```python
from build123d import *

# Parameters (mm, degrees)
BOSS_EXTRUDE1_DEPTH = 2.5
SKETCH2_R           = 1.5
CUT_EXTRUDE1_DEPTH  = 10
SKETCH3_R           = 4.25
SKETCH3_R_2         = 2.75
BOSS_EXTRUDE2_DEPTH = 3.5
SKETCH4_R           = 3.75
SKETCH4_R_2         = 3.25
BOSS_EXTRUDE3_DEPTH = 0.5


with BuildPart() as part:
    # Sketch1 → Boss-Extrude1 (new body)
    with BuildSketch(Plane(origin=(0, 0, 0), x_dir=(1, 0, 0), z_dir=(0, 1, 0))):
        with BuildLine():
            Line((10, -4), (17.506131517, -2.448230154))
            ThreePointArc((17.506131517, -2.448230154), (19.5, 0), (17.506131517, 2.448230154))
            Line((17.506131517, 2.448230154), (10, 4))
            Line((10, 4), (3.774917218, 4))
            ThreePointArc((3.774917218, 4), (0, 5.5), (-3.774917218, 4))
            Line((-3.774917218, 4), (-10, 4))
            Line((-10, 4), (-17.506131517, 2.448230154))
            ThreePointArc((-17.506131517, 2.448230154), (-19.5, 0), (-17.506131517, -2.448230154))
            Line((-17.506131517, -2.448230154), (-10, -4))
            Line((-10, -4), (-3.774917218, -4))
            ThreePointArc((-3.774917218, -4), (0, -5.5), (3.774917218, -4))
            Line((3.774917218, -4), (10, -4))
        make_face()
    extrude(amount=BOSS_EXTRUDE1_DEPTH)

    # Sketch2 → Cut-Extrude1 (cut)
    with BuildSketch(Plane(origin=(0, 2.5, 0), x_dir=(1, 0, 0), z_dir=(0, 1, 0))):
        with Locations(Location((0, 0, 0), (0, 0, 270))):
            Circle(SKETCH2_R)
    extrude(amount=-CUT_EXTRUDE1_DEPTH, mode=Mode.SUBTRACT)

    # Sketch3 → Boss-Extrude2 (add)
    with BuildSketch(Plane(origin=(0, 2.5, 0), x_dir=(1, 0, 0), z_dir=(0, 1, 0))):
        with Locations(Location((0, 0, 0), (0, 0, 270))):
            Circle(SKETCH3_R)
        with Locations(Location((0, 0, 0), (0, 0, 270))):
            Circle(SKETCH3_R_2, mode=Mode.SUBTRACT)
    extrude(amount=BOSS_EXTRUDE2_DEPTH)

    # Sketch4 → Boss-Extrude3 (add)
    with BuildSketch(Plane.XZ):
        with Locations(Location((0, 0, 0), (0, 0, 90))):
            Circle(SKETCH4_R)
        with Locations(Location((0, 0, 0), (0, 0, 270))):
            Circle(SKETCH4_R_2, mode=Mode.SUBTRACT)
    extrude(amount=BOSS_EXTRUDE3_DEPTH)


solid = part.part
```
Geometry check sheet. Reference: the model listing, model coordinates, mm. A direction names the side the tool comes from. Round coordinates to 2 decimals unless told otherwise and drop trailing zeros. Loops run counter-clockwise (first coordinate to the right, second up) from the corner with the lowest first, then second, coordinate; pieces in that order, holes last. Notation, with made-up numbers: (14, -17) - (53, -17) arc R36 cw to (53, 22) - close; hole circle Ø6 at (28, -28). An arc over 180 degrees is marked (long way). Write each question's results on one line, items separated by ' | '. Start each with the question number.
Q1. Cross-section at A-A on z = 0. Enter the section's corners in (x, y), and give its area (3 significant figures).
Q2. Thickness scan on line 1 (X direction, y = 4.65, z = 0); line 2 (X direction, y = -0.3, z = 0); line 3 (Y direction, x = 10, z = 3). Record the ranges inside material, lowest first. Write a range as [from, to].
Q3. Cross-section at B-B on y = 0.75. Enter the section's corners in (x, z).
Q4. Access from +Z, -Z, +X, -X, +Y, -Y to the whole of each face (thin tool, end or side, straight path). Record for faces 5 (the cylindrical face through (4.214, 4.226, -0.553)), 6 (the flat face through (7, 1, -4)), 7 (the flat face through (7, 1, 4)).
Q5. Gauge pin test, flat ends, axial feed: P1, Ø1.2, axis at x = 5.5, y = 1.5, coming from the -Z side; P2, Ø3, axis at x = -7, y = 1.5, coming from the +Z side; P3, Ø1.5, axis at x = -3, y = 2.5, coming from the -Z side. Record the tip position at first contact, or that the pin passes through.
Q6. Cross-section at D-D on y = 4.25. Enter the section's corners in (x, z).
Q7. Release check for a two-part mould opening along X. For faces 1 (the cylindrical face through (-0.165, -0.246, -3.746)), 2 (the flat face through (13.701, 1.232, 3.235)), 3 (the cylindrical face through (-2.685, 4.226, -0.596)), 4 (the flat face through (-7, 1, 4)) record: +X half, -X half, draft (parallel to the pull), parting line (faces both ways), or undercut.
Q8. Cross-section at C-C on x = 0. Enter the section's corners in (y, z), and give its area (3 significant figures).
Answers below:
1) outline: (-19.5, 0) - (-3.75, 0) - (-3.75, -0.5) - (-3.25, -0.5) - (-3.25, 0) - (-1.5, 0) - (-1.5, 2.5) - (-2.75, 2.5) - (-2.75, 6) - (-4.25, 6) - (-4.25, 2.5) - (-19.5, 2.5) - close; (1.5, 0) - (3.25, 0) - (3.25, -0.5) - (3.75, -0.5) - (3.75, 0) - (19.5, 0) - (19.5, 2.5) - (4.25, 2.5) - (4.25, 6) - (2.75, 6) - (2.75, 2.5) - (1.5, 2.5) - close | area: 101 mm²
2) line 1: x = [-4.25, -2.75], [2.75, 4.25] | line 2: x = [-3.75, -3.25], [3.25, 3.75] | line 3: y = [0, 2.5]
3) outline: (-17.51, -2.45) - (-10, -4) - (-3.77, -4) arc R5.5 ccw to (3.77, -4) - (10, -4) - (17.51, -2.45) arc R2.5 ccw to (17.51, 2.45) - (10, 4) - (3.77, 4) arc R5.5 ccw to (-3.77, 4) - (-10, 4) - (-17.51, 2.45) arc R2.5 ccw to start; hole circle Ø3 at (0, 0)
4) face 5: +Y | face 6: -Z, +X, +Y, -Y | face 7: +Z, +X, +Y, -Y
5) P1: stops at z = -4 | P2: stops at z = 4 | P3: stops at z = -5.02
6) outline: circle Ø8.5 at (0, 0); hole circle Ø5.5 at (0, 0)
7) face 1: parting line | face 2: +X half | face 3: undercut | face 4: draft
8) outline: (-0.5, -3.75) - (0, -3.75) - (0, -5.5) - (2.5, -5.5) - (2.5, -4.25) - (6, -4.25) - (6, -2.75) - (2.5, -2.75) - (2.5, -1.5) - (0, -1.5) - (0, -3.25) - (-0.5, -3.25) - close; (-0.5, 3.25) - (0, 3.25) - (0, 1.5) - (2.5, 1.5) - (2.5, 2.75) - (6, 2.75) - (6, 4.25) - (2.5, 4.25) - (2.5, 5.5) - (0, 5.5) - (0, 3.75) - (-0.5, 3.75) - close | area: 31.0 mm²
